Geometry check sheet. Reference: the model listing, model coordinates, mm. Face numbers are marked on the shaded views. Coordinates: 2 decimals unless noted, no trailing zeros. Order: outer loops, then holes, each group sorted by start corner. A loop starts at its lowest first (then second) coordinate and runs counter-clockwise, first axis right, second up. Notation, with made-up numbers: (-26.75, -19.75) - (7.25, -19.75) arc R18 cw to (7.25, 11.25) - close; hole circle Ø3 at (7.25, 67.25). An arc over 180 degrees is marked (long way). Return JSON: item names as keys, results as strings. Group by question number.
Item 1: Scan lines: probe 1 along Y at (x, z) = (-3, 0); probe 2 along X at (y, z) = (-2.4, 0); probe 3 along Z at (x, y) = (1.25, -1.45). Record each from-to range of solid material in increasing order.
Item 2: Gauge pin test, flat end, axial feed: pin 1 (2 mm diameter, centred on x = 0, y = 0, fed in from +Z). Record the tip position at first contact, or that the pin passes through.
Item 3: Draft check along Y on the marked faces 1, 2, 3 and 4. Enter one of: pulls with the +Y half, pulls with the -Y half, needs draft (parallel to the pull), parting line crosses it, or undercut.
Item 4: Section check D-D on y = -2.15. Enter the section's corners in (x, z), then the cut area to 3 significant figures.
Item 5: Section check C-C on z = -3.5. Enter the section's corners in (x, y).
Item 6: Section check B-B on z = 0. Enter the section's corners in (x, y), then the cut area to 4 significant figures.
Item 7: Section check A-A on x = 0. Enter the section's corners in (y, z).
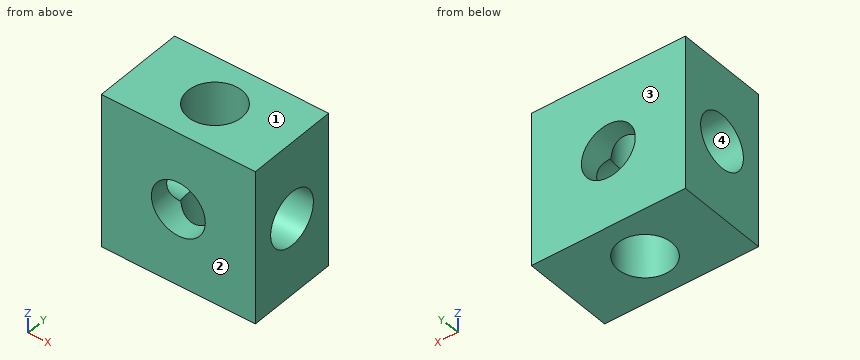
from build123d import *

# Parameters (mm, degrees)
SKETCH_1_W          = 10
SKETCH_1_H          = 10
SKETCH_1_R          = 1.75
EXTRUDE_1_DEPTH     = 3
SKETCH_3_R          = 1.75
CUT_EXTRUDE_1_DEPTH = 8.5
SKETCH_4_R          = 1.75
CUT_EXTRUDE_2_DEPTH = 8.5


with BuildPart() as part:
    # 草图1 → 凸台-拉伸1 (new body, symmetric)
    with BuildSketch(Plane(origin=(0, 0, 0), x_dir=(1, 0, 0), z_dir=(0, 1, 0))):
        Rectangle(SKETCH_1_W, SKETCH_1_H)
        Circle(SKETCH_1_R, mode=Mode.SUBTRACT)
    extrude(amount=EXTRUDE_1_DEPTH, both=True)

    # 草图3 → 切除-拉伸1 (cut, symmetric)
    with BuildSketch(Plane.XY):
        Circle(SKETCH_3_R)
    extrude(amount=CUT_EXTRUDE_1_DEPTH, both=True, mode=Mode.SUBTRACT)

    # 草图4 → 切除-拉伸2 (cut, symmetric)
    with BuildSketch(Plane(origin=(0, 0, 0), x_dir=(0, 0, -1), z_dir=(1, 0, 0))):
        Circle(SKETCH_4_R)
    extrude(amount=CUT_EXTRUDE_2_DEPTH, both=True, mode=Mode.SUBTRACT)


solid = part.part
Computed:
{
 "1": {"probe 1": "y = -3 to -1.75, 1.75 to 3", "probe 2": "x = -5 to -1.75, 1.75 to 5", "probe 3": "z = -5 to -1.22, 1.22 to 5"},
 "2": {"pin 1": "passes through"},
 "3": {"face 1": "needs draft", "face 2": "pulls with the -Y half", "face 3": "pulls with the +Y half", "face 4": "undercut"},
 "4": {"outline": "(-5, -5) - (5, -5) - (5, 5) - (-5, 5) - close; hole circle Ø3.5 at (0, 0)", "area": "90.4 mm²"},
 "5": {"outline": "(-5, -3) - (5, -3) - (5, 3) - (-5, 3) - close; hole circle Ø3.5 at (0, 0)"},
 "6": {"outline": "(-5, -3) - (-1.75, -3) - (-1.75, -1.75) - (-5, -1.75) - close; (-5, 1.75) - (-1.75, 1.75) - (-1.75, 3) - (-5, 3) - close; (1.75, -3) - (5, -3) - (5, -1.75) - (1.75, -1.75) - close; (1.75, 1.75) - (5, 1.75) - (5, 3) - (1.75, 3) - close", "area": "16.25 mm²"},
 "7": {"outline": "(-3, -5) - (-1.75, -5) - (-1.75, -1.75) - (-3, -1.75) - close; (-3, 1.75) - (-1.75, 1.75) - (-1.75, 5) - (-3, 5) - close; (1.75, -5) - (3, -5) - (3, -1.75) - (1.75, -1.75) - close; (1.75, 1.75) - (3, 1.75) - (3, 5) - (1.75, 5) - close"}
}
